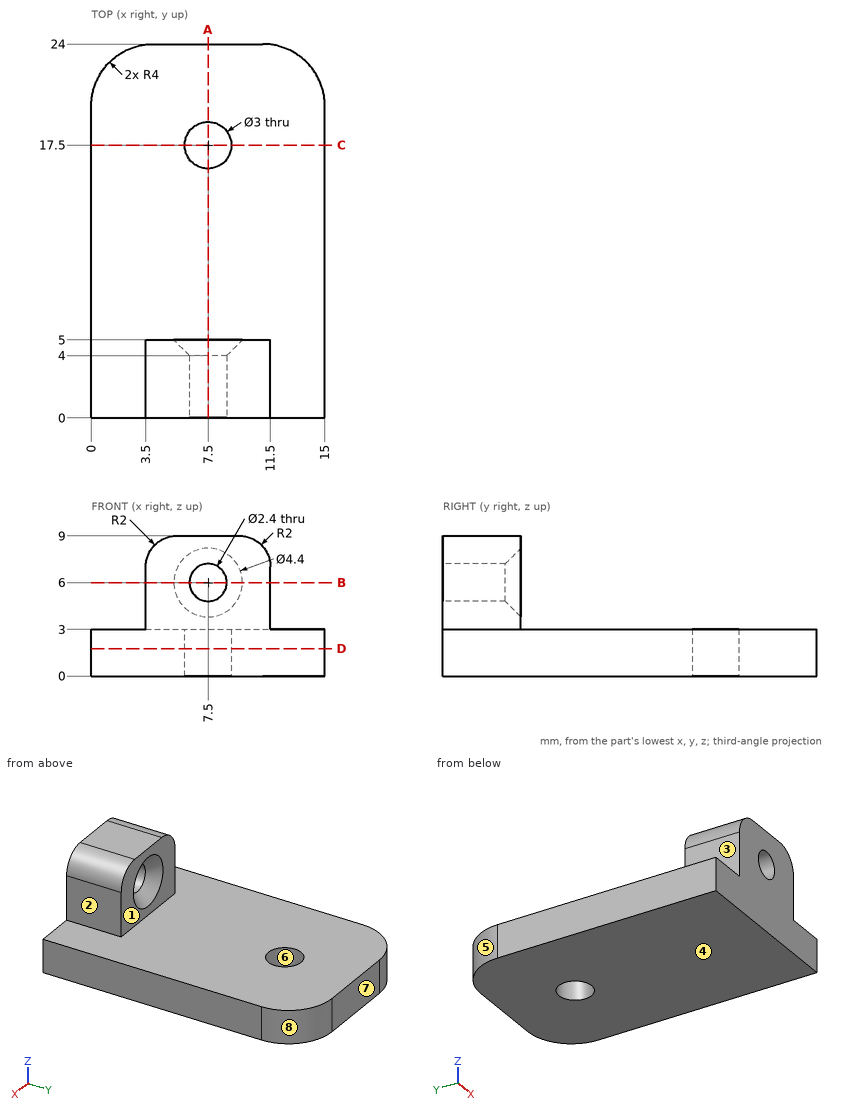
Here's the drawing with two shaded views (mm, measured from the low corner). I have some questions. A direction names the side the tool comes from. Give positions to 0.01 mm unless a question says otherwise; leave off trailing zeros. Order: outer loops, then holes, each group sorted by start corner. A loop starts at its lowest first (then second) coordinate and runs counter-clockwise, first axis right, second up. Notation, with made-up numbers: (-8.5, 40.5) -> (30.5, 40.5) arc R35 ccw to (30.5, 79.5) -> close; hole circle Ø4 at (-8.5, 47). An arc over 180 degrees is marked (long way). Use a Markdown table: item, result. Add a question column.
Item 1: If we mould it in two halves opening along X, with no side actions, what happens to the marked faces 6, 7 and 8? For each: pulls with the +X half, pulls with the -X half, needs draft (parallel to the pull), parting line crosses it, or undercut.
Item 2: I need wall thicknesses on line 1 (X direction, y = 1.15, z = 6); line 2 (Y direction, x = 7.5, z = 0.65); line 3 (Z direction, x = 6, y = 9.75). Which ranges of each line are inside material? Lowest first, please.
Item 3: Imagine slicing it at B-B on z = 6. Please give me the cut outline in (x, y).
Item 4: Will these pins go through, and if not, where does the flat tip stop? pin 1 (2 mm diameter, centred on y = 1.5, z = 5, fed in from -X); pin 2 (3 mm diameter, centred on x = 3.5, y = 18.5, fed in from -Z); pin 3 (2 mm diameter, centred on y = 2.5, z = 6, fed in from +X); pin 4 (3 mm diameter, centred on x = 7.5, z = 6, fed in from +Y).
Item 5: Imagine slicing it at D-D on z = 1.75. Please give me the cut outline in (x, y).
Item 6: Imagine slicing it at A-A on x = 7.5. Please give me the cut outline in (y, z), plus the area to 3 significant figures.
Item 7: Imagine slicing it at C-C on y = 17.5. Please give me the cut outline in (x, z), plus the area to 3 significant figures.
Item 8: For the marked faces 1, 2, 3, 4 and 5, which set-ups out of +Z, -Z, +X, -X, +Y, -Y let a thin tool reach every point of the face, with its end or its side?
Data:
| question | item | result |
|---|---|---|
| 1 | face 6 | undercut |
| 1 | face 7 | needs draft |
| 1 | face 8 | pulls with the +X half |
| 2 | line 1 | x = 3.5 to 6.3, 8.7 to 11.5 |
| 2 | line 2 | y = 0 to 16, 19 to 24 |
| 2 | line 3 | z = 0 to 3 |
| 3 | outline | (3.5, 0) -> (6.3, 0) -> (6.3, 4) -> (5.3, 5) -> (3.5, 5) -> close; (8.7, 0) -> (11.5, 0) -> (11.5, 5) -> (9.7, 5) -> (8.7, 4) -> close |
| 4 | pin 1 | stops at x = 3.5 |
| 4 | pin 2 | stops at z = 0 |
| 4 | pin 3 | stops at x = 11.5 |
| 4 | pin 4 | stops at y = 4.3 |
| 5 | outline | (0, 0) -> (15, 0) -> (15, 20) arc R4 ccw to (11, 24) -> (4, 24) arc R4 ccw to (0, 20) -> close; hole circle Ø3 at (7.5, 17.5) |
| 6 | outline | (0, 0) -> (16, 0) -> (16, 3) -> (5, 3) -> (5, 3.8) -> (4, 4.8) -> (0, 4.8) -> close; (0, 7.2) -> (4, 7.2) -> (5, 8.2) -> (5, 9) -> (0, 9) -> close; (19, 0) -> (24, 0) -> (24, 3) -> (19, 3) -> close |
| 6 | area | 80.0 mm² |
| 7 | outline | (0, 0) -> (6, 0) -> (6, 3) -> (0, 3) -> close; (9, 0) -> (15, 0) -> (15, 3) -> (9, 3) -> close |
| 7 | area | 36.0 mm² |
| 8 | face 1 | +Z, +X, -X, +Y |
| 8 | face 2 | +Z, +X, +Y, -Y |
| 8 | face 3 | +Z, -X, +Y, -Y |
| 8 | face 4 | -Z, +X, -X, +Y, -Y |
| 8 | face 5 | +Z, -Z, -X, +Y |
